Work out the finished part from the listing and answer in its coordinate system (mm). A direction names the side the tool comes from. Coordinates: 2 decimals unless noted, no trailing zeros. Order: outer loops, then holes, each group sorted by start corner. A loop starts at its lowest first (then second) coordinate and runs counter-clockwise, first axis right, second up. Notation, with made-up numbers: M 63.5,-22.75 L 122.5,-22.75 A15 ccw 122.5,-18.75 Z; hole C 59,63.25 d3. An arc over 180 degrees is marked long. Write item = value, one per line. Start each with the question number.
Q1. Find section B-B on x = 155. Give the vertices of the cut face in (y, z) (3 decimals).
Q2. Find section C-C on y = 63. Give the vertices of the cut face in (x, z), and give its area (3 significant figures).
Q3. Each of these flat-tipped pins is pushed along its axis until it touches: P1, Ø8, axis at x = 85, z = 6, coming from the +Y side; P2, Ø7.5, axis at x = 135, y = 84, coming from the -Z side; P3, Ø2, axis at x = -31.5, z = 10.5, coming from the -Y side; P4, Ø3, axis at x = 67, z = 3.5, coming from the -Y side. Where does it stop, or does it pass through?
Q4. A tool of negligible diameter and unlimited length cuts with its end or side. For faces 1 (the flat face through (-72.5, 188, 8)), 2 (the cylindrical face through (63.3, 194.4, 8.4)), from which of +Z, -Z, +X, -X, +Y, -Y can it reach the whole face along a straight path? Write none if from no direction.
Q5. Straight lines are drawn through the part: line 1 along Y through (x, z) = (0, 11); line 2 along Y through (x, z) = (58, 13.5); line 3 along X through (y, z) = (65.5, 1.75). For each, find the intervals that lie inside material, in ascending order.
Q6. Determine the mould class of faces 3 (the cylindrical face through (7.07, -186.33, 8.38)), 4 (the cylindrical face through (-56.7, 194.4, 8.4)), 5 (the flat face through (85, -30, 17)), 6 (the cylindrical face through (133.062, 80.274, 8.381)) for opening direction X: released by +X, released by -X, zero draft, split by the parting line, or undercut.
Q7. Find section A-A on y = 0. Give the vertices of the cut face in (x, z).
Q8. Find section D-D on z = 4. Give the number of separate pieces and of enclosed holes in the cut face, and give its area (3 significant figures).
```python
from build123d import *

# Parameters (mm, degrees)
SKETCH1_R                   = 4.5
SKETCH1_R_2                 = 4
SKETCH1_R_3                 = 3.5
SKETCH1_R_4                 = 87.5
BOSS_EXTRUDE1_DEPTH         = 17
F_3_8_CLEARANCE_HOLE1_D     = 9.8044
F_3_8_CLEARANCE_HOLE1_DEPTH = 51.26
F_3_8_CLEARANCE_HOLE1_TIP   = 2.945538927
M10_CLEARANCE_HOLE1_D       = 10.5
M10_CLEARANCE_HOLE1_DEPTH   = 51.26
M10_CLEARANCE_HOLE1_TIP     = 3.15451825
M8_CLEARANCE_HOLE1_D        = 8.4
M8_CLEARANCE_HOLE1_DEPTH    = 51.26
M8_CLEARANCE_HOLE1_TIP      = 2.5236146


with BuildPart() as part:
    # Sketch1 → Boss-Extrude1 (new body)
    with BuildSketch(Plane.XY):
        with BuildLine():
            Line((-60, 209.5), (60, 209.5))
            ThreePointArc((60, 209.5), (68.838834765, 205.838834765), (72.5, 197))
            Line((72.5, 197), (72.5, 178.304283367))
            ThreePointArc((72.5, 178.304283367), (74.07408405, 172.918752715), (78.30078808, 169.228677643))
            ThreePointArc((78.30078808, 169.228677643), (0, -186.465435807), (-78.30078808, 169.228677643))
            ThreePointArc((-78.30078808, 169.228677643), (-74.07408405, 172.918752715), (-72.5, 178.304283367))
            Line((-72.5, 178.304283367), (-72.5, 197))
            ThreePointArc((-72.5, 197), (-68.838834765, 205.838834765), (-60, 209.5))
        make_face()
        with Locations((-84, 143)):
            Circle(SKETCH1_R, mode=Mode.SUBTRACT)
        with Locations((-60, 197)):
            Circle(SKETCH1_R_2, mode=Mode.SUBTRACT)
        with Locations((60, 197)):
            Circle(SKETCH1_R_3, mode=Mode.SUBTRACT)
        with Locations((135, 84)):
            Circle(SKETCH1_R_3, mode=Mode.SUBTRACT)
        with Locations((155, -45)):
            Circle(SKETCH1_R, mode=Mode.SUBTRACT)
        with Locations((-155, -45)):
            Circle(SKETCH1_R, mode=Mode.SUBTRACT)
        Circle(SKETCH1_R_4, mode=Mode.SUBTRACT)
        with Locations((-153, 63)):
            Circle(SKETCH1_R, mode=Mode.SUBTRACT)
    extrude(amount=BOSS_EXTRUDE1_DEPTH)

    # 3/8 Clearance Hole1
    with Locations(Plane(origin=(75.50716213, 75.50716213, 17), x_dir=(1, 0, 0), z_dir=(0, 0, 1))):
        with Locations((0, 0), (0, -151.01432426), (-151.01432426, -151.01432426), (-151.01432426, 0), (-75.50716213, 31.17283787), (31.17283787, -75.50716213), (-182.18716213, -75.50716213), (-75.50716213, -182.18716213)):
            Hole(F_3_8_CLEARANCE_HOLE1_D / 2, depth=F_3_8_CLEARANCE_HOLE1_DEPTH)
            with Locations((0, 0, -(F_3_8_CLEARANCE_HOLE1_DEPTH + F_3_8_CLEARANCE_HOLE1_TIP / 2))):  # 118° drill point
                Cone(0, F_3_8_CLEARANCE_HOLE1_D / 2, F_3_8_CLEARANCE_HOLE1_TIP, mode=Mode.SUBTRACT)

    # M10 Clearance Hole1
    with Locations(Plane(origin=(155, -45, 17), x_dir=(1, 0, 0), z_dir=(0, 0, 1))):
        with Locations((0, 0), (-310, 0), (-308, 108), (-239, 188)):
            Hole(M10_CLEARANCE_HOLE1_D / 2, depth=M10_CLEARANCE_HOLE1_DEPTH)
            with Locations((0, 0, -(M10_CLEARANCE_HOLE1_DEPTH + M10_CLEARANCE_HOLE1_TIP / 2))):  # 118° drill point
                Cone(0, M10_CLEARANCE_HOLE1_D / 2, M10_CLEARANCE_HOLE1_TIP, mode=Mode.SUBTRACT)

    # M8 Clearance Hole1
    with Locations(Plane(origin=(-60, 197, 17), x_dir=(1, 0, 0), z_dir=(0, 0, 1))):
        with Locations((0, 0), (120, 0), (195, -113)):
            Hole(M8_CLEARANCE_HOLE1_D / 2, depth=M8_CLEARANCE_HOLE1_DEPTH)
            with Locations((0, 0, -(M8_CLEARANCE_HOLE1_DEPTH + M8_CLEARANCE_HOLE1_TIP / 2))):  # 118° drill point
                Cone(0, M8_CLEARANCE_HOLE1_D / 2, M8_CLEARANCE_HOLE1_TIP, mode=Mode.SUBTRACT)


solid = part.part
```
Findings below:
q1.outline = M -103.655,0 L -50.25,0 L -50.25,17 L -103.655,17 Z; M -39.75,0 L 103.655,0 L 103.655,17 L -39.75,17 Z
q2.outline = M -175.5,0 L -158.25,0 L -158.25,17 L -175.5,17 Z; M -147.75,0 L -60.72,0 L -60.72,17 L -147.75,17 Z; M 60.72,0 L 175.5,0 L 175.5,17 L 60.72,17 Z
q2.area = 3,720 mm^2
q3.P1 = 167.95
q3.P2 = through
q3.P3 = -183.95
q3.P4 = -174.58
q4.face_1 = +Z, -Z, -X, +Y
q4.face_2 = +Z, -Z
q5.line_1 = -186.47 to -111.58, -101.78 to -87.5, 87.5 to 101.78, 111.58 to 209.5
q5.line_2 = -177.22 to -65.52, 65.52 to 193.31, 200.69 to 209.5
q5.line_3 = -174.58 to -157.62, -148.38 to -58.02, 58.02 to 174.58
q6.face_3 = split by the parting line
q6.face_4 = undercut
q6.face_5 = zero draft
q6.face_6 = undercut
q7.outline = M -186.47,0 L -111.58,0 L -111.58,17 L -186.47,17 Z; M -101.78,0 L -87.5,0 L -87.5,17 L -101.78,17 Z; M 87.5,0 L 101.78,0 L 101.78,17 L 87.5,17 Z; M 111.58,0 L 186.47,0 L 186.47,17 L 111.58,17 Z
q8.separate_pieces = 1
q8.enclosed_holes = 16
q8.area = 88,000 mm^2
